Could you check a few things on this model? Use its own coordinates, in mm. A direction names the side the tool comes from. Round coordinates to 2 decimals unless told otherwise and drop trailing zeros. Write each loop counter-clockwise with the first axis right and the second up, starting at its lowest first coordinate (ties: lowest second). Pieces come first, ordered by that corner, then holes.
```python
from build123d import *

# Parameters (mm, degrees)
PAD006_DEPTH = 10
FILLET001_R  = 3
PAD010_DEPTH = 4


with BuildPart() as part:
    # Sketch006 → Pad006 (new body)
    with BuildSketch(Plane.XZ):
        with BuildLine():
            Line((18.25, 57), (12.25, 57))
            Line((12.25, 57), (0, 0))
            Line((0, 0), (50, 0))
            Line((50, 0), (37.75, 57))
            Line((37.75, 57), (31.75, 57))
            Line((30.75, 42.535534), (31.75, 57))
            ThreePointArc((31.75, 39), (31.495191, 40.837117), (30.75, 42.535534))
            Line((31.75, 8.5), (31.75, 39))
            ThreePointArc((18.25, 8.5), (25, 7), (31.75, 8.5))
            Line((18.25, 39), (18.25, 8.5))
            ThreePointArc((19.25, 42.535534), (18.504809, 40.837117), (18.25, 39))
            Line((19.25, 42.535534), (18.25, 57))
        make_face()
    extrude(amount=-PAD006_DEPTH)

    # Fillet001
    fillet001_edges = [part.edges().sort_by_distance(p)[0] for p in [
        (31.75, 10, 23.75),
        (18.25, 10, 23.75),
    ]]
    fillet(fillet001_edges, radius=FILLET001_R)

    # Sketch009 → Pad010 (join)
    with BuildSketch(Plane.XZ):
        Polygon((11, -4), (11, 5.262975), (39, 5.262975), (39, -4), (35, -4), (35, 0), (15, 0), (15, -4), align=None)
    extrude(amount=-PAD010_DEPTH)


solid = part.part
```
Q1. I'm going to push flat-ended pins straight in: pin 1 Ø5 at (y, z) = (1, 3.5) entering from -X; pin 2 Ø3.5 at (y, z) = (3, 16.5) entering from +X; pin 3 Ø4 at (y, z) = (1, 43) entering from +X. Where does each tip first touch, or does it pass through?
Q2. Imagine slicing it at A-A, the plane z = 35. Write out the boundary of the cut face in (x, y), then the cut area to 3 significant figures.
Q3. If I drill on L1, parallel to Z at x = 16, y = 1.5; L2, parallel to X at y = 8.5, z = 21; L3, parallel to X at y = 3, z = 19, over which ranges is the centre line in solid material (lowest first)?
Q4. On a 3-axis mill with a long thin cutter (end or side, diameter ignored), from which of +Z, -Z, +X, -X, +Y, -Y can I reach the whole of each face in a straight line? I mean faces 5 (the flat face through (31.75, 3, 24)), 6 (the flat face through (15, 2, -2)), 7 (the cylindrical face through (17.39, 9.1, 23.54)). Say none if no direction works.
Q5. Imagine slicing it at D-D, the plane x = 22.5. Write out the boundary of the cut face in (y, z).
Q6. We'd pull the mould along Z, two halves only. Please class faces 1 (the flat face through (14, 0, 20)), 2 (the flat face through (13, 2, -4)), 3 (the cylindrical face through (18.51, 3.45, 40.86)), 4 (the flat face through (18.757, 4.93, 49.667)): pulls with the +Z half, pulls with the -Z half, needs draft (parallel to the pull), parting line crosses it, or undercut.
Q7. Imagine slicing it at C-C, the plane z = 21.5. Write out the boundary of the cut face in (x, y).
Results found:
1. pin 1: stops at x = 0.21
1. pin 2: stops at x = 46.83
1. pin 3: stops at x = 41.19
2. outline: (7.52, 0) - (18.25, 0) - (18.25, 7) arc R3 ccw to (15.25, 10) - (7.52, 10) - close; (31.75, 0) - (42.48, 0) - (42.48, 10) - (34.75, 10) arc R3 ccw to (31.75, 7) - close
2. area: 211 mm2
3. L1: z = 0 to 57
3. L2: x = 4.51 to 17.85, 32.15 to 45.49
3. L3: x = 4.08 to 18.25, 31.75 to 45.92
4. face 5: +Y, -Y
4. face 6: -Z, +Y, -Y
4. face 7: +Y
5. outline: (0, 0) - (10, 0) - (10, 7.2) - (0, 7.2) - close
6. face 1: needs draft
6. face 2: pulls with the -Z half
6. face 3: undercut
6. face 4: pulls with the +Z half
7. outline: (4.62, 0) - (18.25, 0) - (18.25, 7) arc R3 ccw to (15.25, 10) - (4.62, 10) - close; (31.75, 0) - (45.38, 0) - (45.38, 10) - (34.75, 10) arc R3 ccw to (31.75, 7) - close
